Study the drawing (mm; zero at the part's minimum x, y, z) and answer. A direction names the side the tool comes from. Round coordinates to 2 decimals unless told otherwise and drop trailing zeros. Write each loop counter-clockwise with the first axis right and the second up, starting at its lowest first coordinate (ties: lowest second). Pieces come first, ordered by that corner, then holes.
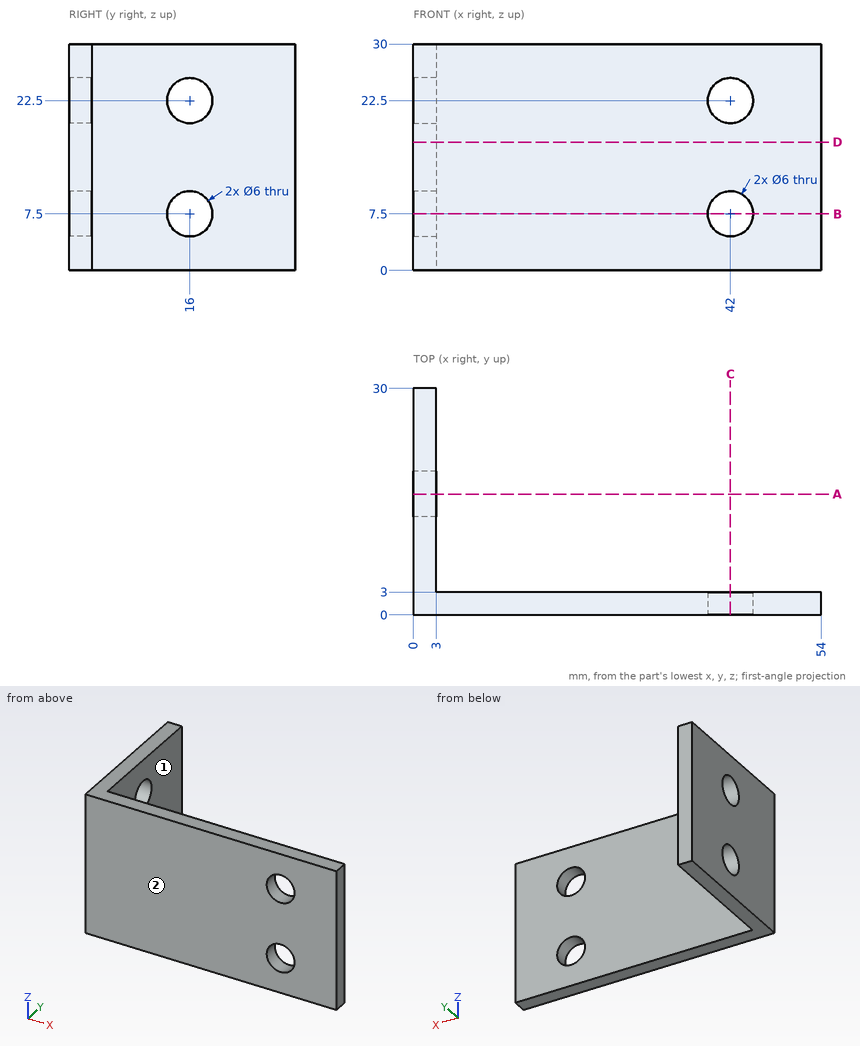
Q1. Find the intervals of material crossed by L1, parallel to Z at x = 42, y = 2.15; L2, parallel to X at y = 1.6, z = 22.5; L3, parallel to Y at x = 45, z = 3.25, in increasing order.
Q2. Find section D-D (z = 17). Determine the outline of the cut face in (x, y).
Q3. Given pin 1 (5 mm diameter, centred on x = 42, z = 22.5, fed in from +Y); pin 2 (2 mm diameter, centred on y = 13.5, z = 26.5, fed in from +X); pin 3 (3 mm diameter, centred on x = 35.5, z = 24, fed in from +Y), each flat-ended and moving along its own axis, determine where each tip first touches the part or whether it passes through.
Q4. A tool of negligible diameter and unlimited length cuts with its end or side. For the marked faces 1 and 2, from which of +Z, -Z, +X, -X, +Y, -Y can it reach the whole face along a straight path? Write none if from no direction.
Q5. Find section A-A (y = 16). Determine the outline of the cut face in (x, z), plus the area to 3 significant figures.
Q6. Find section B-B (z = 7.5). Determine the outline of the cut face in (x, y), plus the area to 3 significant figures.
Report:
1. L1: z = 0 to 4.5, 10.5 to 19.5, 25.5 to 30
1. L2: x = 0 to 39, 45 to 54
1. L3: y = 0 to 3
2. outline: (0, 0) - (54, 0) - (54, 3) - (3, 3) - (3, 30) - (0, 30) - close
3. pin 1: passes through
3. pin 2: stops at x = 3
3. pin 3: stops at y = 3
4. face 1: +Z, -Z, +X, +Y
4. face 2: +Z, -Z, +X, -X, -Y
5. outline: (0, 0) - (3, 0) - (3, 4.5) - (0, 4.5) - close; (0, 10.5) - (3, 10.5) - (3, 19.5) - (0, 19.5) - close; (0, 25.5) - (3, 25.5) - (3, 30) - (0, 30) - close
5. area: 54.0 mm2
6. outline: (0, 0) - (39, 0) - (39, 3) - (3, 3) - (3, 13) - (0, 13) - close; (0, 19) - (3, 19) - (3, 30) - (0, 30) - close; (45, 0) - (54, 0) - (54, 3) - (45, 3) - close
6. area: 207 mm2
